Here's how the part is built. I have some questions about the finished solid (model axes, mm). A direction names the side the tool comes from. Give positions to 0.01 mm unless a question says otherwise; leave off trailing zeros. Write each loop counter-clockwise with the first axis right and the second up, starting at its lowest first coordinate (ties: lowest second). Pieces come first, ordered by that corner, then holes. Notation, with made-up numbers: M 25,-26.75 L 45,-26.75 A13 cw 45,-12.75 Z; hole C 7.25,63 d4. An arc over 180 degrees is marked long. Use one line per item in the form item = value. Start each with the question number.
from build123d import *

# Parameters (mm, degrees)
SKETCH_1_R          = 12.1
EXTRUDE_1_DEPTH     = 7
FILLET_3_R          = 7
EXTRUDE_START       = -1.9
SKETCH_7_R          = 12.1
SKETCH_7_R_2        = 11.6
EXTRUDE_2_DEPTH     = 1.9
HOLE_WIZARD_M53_D   = 5.5
HOLE_WIZARD_M54_D   = 5.5
CUT_EXTRUDE_1_DEPTH = 3.5


with BuildPart() as part:
    # Эскиз1 → Бобышка-Вытянуть1 (new body)
    with BuildSketch(Plane.XY):
        with BuildLine():
            Line((-9.282257481, -15.602398743), (-25.265839773, -14.994950265))
            ThreePointArc((-25.265839773, -14.994950265), (-30.042860221, -12.854849204), (-32, -8))
            Line((-32, -8), (-32, 15))
            Line((-32, 15), (-8, 15))
            ThreePointArc((-8, 15), (0, 17), (8, 15))
            Line((8, 15), (32, 15))
            Line((32, 15), (32, -8))
            ThreePointArc((32, -8), (30.042860221, -12.854849204), (25.265839773, -14.994950265))
            Line((25.265839773, -14.994950265), (9.282257481, -15.602398743))
            ThreePointArc((9.282257481, -15.602398743), (7.964469385, -15.770214084), (6.696960066, -16.167891819))
            ThreePointArc((6.696960066, -16.167891819), (0, -17.5), (-6.696960066, -16.167891819))
            ThreePointArc((-6.696960066, -16.167891819), (-7.964469385, -15.770214084), (-9.282257481, -15.602398743))
        make_face()
        Circle(SKETCH_1_R, mode=Mode.SUBTRACT)
    extrude(amount=EXTRUDE_1_DEPTH)

    # Скругление3
    fillet_3_edges = [part.edges().sort_by_distance(p)[0] for p in [
        (-32, 15, 3.5),
        (-8, 15, 3.5),
        (8, 15, 3.5),
        (32, 15, 3.5),
    ]]
    fillet(fillet_3_edges, radius=FILLET_3_R)

    # Эскиз7 → Бобышка-Вытянуть2 (add)
    with BuildSketch(Plane.XY.offset(7).offset(EXTRUDE_START)):
        with Locations(Location((0, 0, 0), (0, 0, 90))):
            Circle(SKETCH_7_R)
        Circle(SKETCH_7_R_2, mode=Mode.SUBTRACT)
    extrude(amount=EXTRUDE_2_DEPTH)

    # Отверстие с зазором M53 (through all)
    with Locations(Plane.XY.offset(7)):
        with Locations((-25, 8), (25, 8)):
            Hole(HOLE_WIZARD_M53_D / 2)

    # Отверстие с зазором M54 (through all)
    with Locations(Plane(origin=(-20.850360387, 7.199740636, 7), x_dir=(-1, 0, 0), z_dir=(0, 0, 1))):
        with Locations((-45.850360387, 15.199740636), (4.149639613, 15.199740636)):
            Hole(HOLE_WIZARD_M54_D / 2)

    # Эскиз18 → Вырез-Вытянуть1 (cut)
    with BuildSketch(Plane(origin=(0, 0, 7), x_dir=(1, 0, 0), z_dir=(0, 0, -1))):
        Polygon((20.092522712, -8), (22.546261356, -12.25), (27.453738644, -12.25), (29.907477288, -8), (27.453738644, -3.75), (22.546261356, -3.75), align=None)
        Polygon((-27.453738644, -3.75), (-29.907477288, -8), (-27.453738644, -12.25), (-22.546261356, -12.25), (-20.092522712, -8), (-22.546261356, -3.75), align=None)
        Polygon((20.092522712, 8), (22.546261356, 12.25), (27.453738644, 12.25), (29.907477288, 8), (27.453738644, 3.75), (22.546261356, 3.75), align=None)
        Polygon((-22.546261356, 12.25), (-20.092522712, 8), (-22.546261356, 3.75), (-27.453738644, 3.75), (-29.907477288, 8), (-27.453738644, 12.25), align=None)
    extrude(amount=CUT_EXTRUDE_1_DEPTH, mode=Mode.SUBTRACT)


solid = part.part
1) Suppose I cut it at B-B, the plane y = 0. List the corners of the cut face in (x, z) for me, and give its area (4 significant figures).
2) Suppose I cut it at D-D, the plane y = 6.5. List the corners of the cut face in (x, z) for me, and give its area (3 significant figures).
3) On a 3-axis mill with a long thin cutter (end or side, diameter ignored), from which of +Z, -Z, +X, -X, +Y, -Y can I reach the whole of each face in a straight line? I mean faces 1 (the face through (7.983, -15.766, 3.451)), 2 (the face through (17, 15, 3)), 3 (the face through (25, 5, 3.5)). Say none if no direction works.
4) Suppose I cut it at C-C, the plane z = 1.25. List the corners of the cut face in (x, y) for me, and give its area (3 significant figures).
5) Thinking about a two-plate mould opening in Y: for faces 4 (the face through (-21.337, -10.155, 5.274)), 5 (the face through (0, 17, 3)), 6 (the face through (-30, -12.9, 3.5)), which applies, released by +Y, released by -Y, zero draft, split by the parting line, or undercut?
6) Suppose I cut it at A-A, the plane x = 0. List the corners of the cut face in (y, z) for me, and give its area (3 significant figures).
7) Will these pins go through, and if not, where does the flat tip stop? P1, Ø4, axis at x = 24.5, z = 6, coming from the +Y side; P2, Ø1, axis at x = -25, z = 5, coming from the -Y side; P3, Ø2.5, axis at x = -24.5, y = -6, coming from the +Z side.
8) Please list where these lines run through material, in increasing order: line 1 (Y direction, x = -25, z = 2.2); line 2 (X direction, y = -8.5, z = 5.5); line 3 (X direction, y = -5.5, z = 2.5).
Checks:
q1.outline = M -32,0 L -12.1,0 L -12.1,5.1 L -11.6,5.1 L -11.6,7 L -32,7 Z; M 11.6,5.1 L 12.1,5.1 L 12.1,0 L 32,0 L 32,7 L 11.6,7 Z
q1.area = 280.5 mm^2
q2.outline = M -32,0 L -27.3,0 L -27.3,3.5 L -29.04,3.5 L -29.04,7 L -32,7 Z; M -22.7,0 L -10.21,0 L -10.21,5.1 L -9.61,5.1 L -9.61,7 L -20.96,7 L -20.96,3.5 L -22.7,3.5 Z; M 9.61,5.1 L 10.21,5.1 L 10.21,0 L 22.7,0 L 22.7,3.5 L 20.96,3.5 L 20.96,7 L 9.61,7 Z; M 27.3,0 L 32,0 L 32,7 L 29.04,7 L 29.04,3.5 L 27.3,3.5 Z
q2.area = 219 mm^2
q3.face_1 = +Z, -Z, +X, -Y
q3.face_2 = +Z, -Z, +X, +Y
q3.face_3 = +Z
q4.outline = M -32,-8 A7 ccw -25.27,-14.99 L -9.28,-15.6 A7.5 cw -6.7,-16.17 A17.5 ccw 6.7,-16.17 A7.5 cw 9.28,-15.6 L 25.27,-14.99 A7 ccw 32,-8 L 32,8 A7 ccw 25,15 L 9.59,15 A7 cw 6.79,15.58 A17 ccw -6.79,15.58 A7 cw -9.59,15 L -25,15 A7 ccw -32,8 Z; hole C -25,-8 d5.5; hole C -25,8 d5.5; hole C 0,0 d24.2; hole C 25,-8 d5.5; hole C 25,8 d5.5
q4.area = 1,390 mm^2
q5.face_4 = undercut
q5.face_5 = released by +Y
q5.face_6 = released by -Y
q6.outline = M -17.5,0 L -12.1,0 L -12.1,5.1 L -11.6,5.1 L -11.6,7 L -17.5,7 Z; M 11.6,5.1 L 12.1,5.1 L 12.1,0 L 17,0 L 17,7 L 11.6,7 Z
q6.area = 74.0 mm^2
q7.P1 = 15
q7.P2 = -15.02
q7.P3 = 3.5
q8.line_1 = -15.01 to -10.75, -5.25 to 5.25, 10.75 to 15
q8.line_2 = -31.98 to -29.62, -20.38 to -7.89, 7.89 to 20.38, 29.62 to 31.98
q8.line_3 = -32 to -26.15, -23.85 to -10.78, 10.78 to 23.85, 26.15 to 32
